Print and shaded views of the part. All mm, measured from the part's lowest x, y and z. A direction names the side the tool comes from. Round coordinates to 2 decimals unless told otherwise and drop trailing zeros. Loops run counter-clockwise (first coordinate to the right, second up) from the corner with the lowest first, then second, coordinate; pieces in that order, holes last. Notation, with made-up numbers: (12, 67.5) - (40, 67.5) arc R26 ccw to (40, 106.5) - close; hole circle Ø2 at (-36.5, 56). An arc over 180 degrees is marked (long way). Use one line per item in the form item = value.
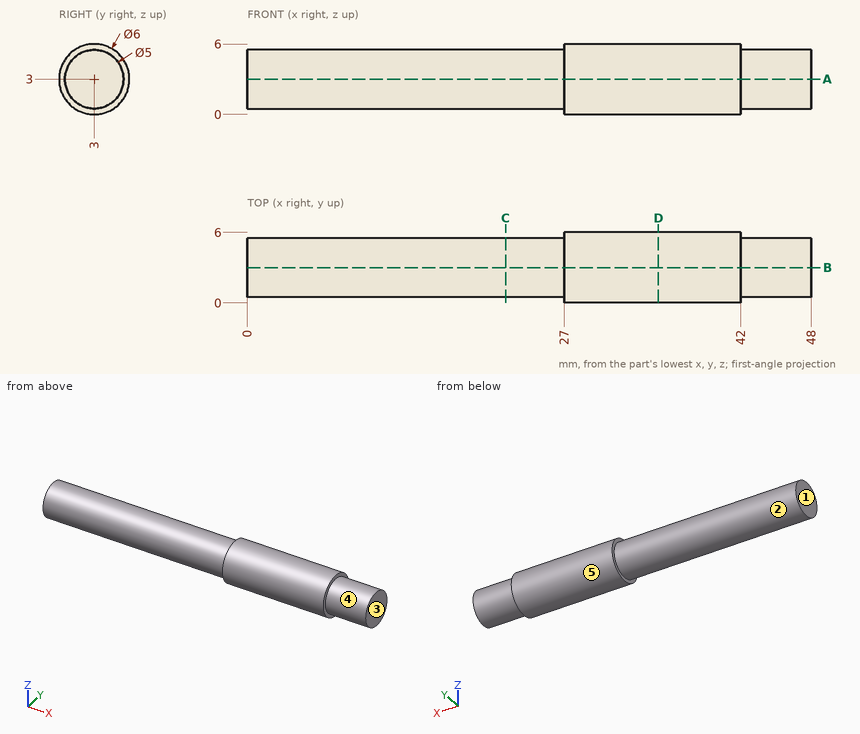
1. Pull direction X, two halves, no side cores. Call the marked faces 1, 2 and 3: +X half, -X half, draft (parallel to the pull), parting line (faces both ways), or undercut.
Geometry check:
face_1 = -X half
face_2 = draft
face_3 = +X half
2. Cut at D-D, the plane x = 35. Give the cut face in (y, z), plus the area to 3 significant figures.
Geometry check:
outline = circle Ø6 at (3, 3)
area = 28.3 mm^2
3. Tool access for the marked faces 4 and 5: list every direction of +Z, -Z, +X, -X, +Y, -Y with a clear straight run to the whole face (end or side of a thin tool).
Geometry check:
face_4 = +X
face_5 = +X, -X
4. Wall check: probe 1 along Y at (x, z) = (6, 3); probe 2 along Z at (x, y) = (5.5, 1.1); probe 3 along Z at (x, y) = (41, 4.85). Give the ranges that are in metal, low to high.
Geometry check:
probe_1 = 0.5 to 5.5
probe_2 = 1.38 to 4.62
probe_3 = 0.64 to 5.36
5. Cut at A-A, the plane z = 3. Give the cut face in (x, y), plus the area to 3 significant figures.
Geometry check:
outline = (0, 0.5) - (27, 0.5) - (27, 0) - (42, 0) - (42, 0.5) - (48, 0.5) - (48, 5.5) - (42, 5.5) - (42, 6) - (27, 6) - (27, 5.5) - (0, 5.5) - close
area = 255 mm^2
6. Cut at C-C, the plane x = 22. Give the cut face in (y, z).
Geometry check:
outline = circle Ø5 at (3, 3)
7. Flat gauge pins, fed straight in: pin 1 (1 mm diameter, centred on x = 35.5, z = 1, fed in from -Y); pin 2 (1.5 mm diameter, centred on x = 40, y = 5, fed in from -Z). Where does each tip first touch, or does it go through?
Geometry check:
pin_1 = 0.4
pin_2 = 0.27
